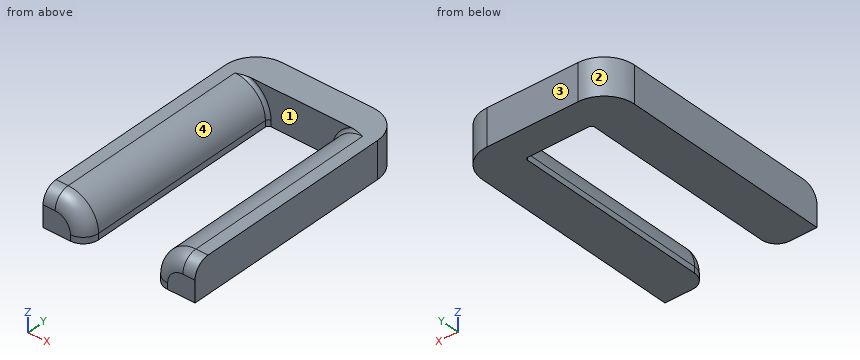
```python
from build123d import *

# Parameters (mm, degrees)
F0_W         = 50
F0_H         = 12
F1_DEPTH     = 10
F2_W         = 14
F2_H         = 12
F3_DEPTH     = 70
F4_R         = 10
F5_R         = 5
F6_T1_DEPTH  = 2
F6_T6_ANGLE  = 132.9890967712
F6_T12_ANGLE = 132.9890967712
F7_R         = 10


# Not quite as in the source:
# - a fillet or chamfer that OpenCascade refuses, or shapes differently, is made with other operations: its cross-section is extruded or revolved along the edge and cut away or added


with BuildPart() as f1:
    # F0 (on Front) → F1 (new body)
    with BuildSketch(Plane.XZ):
        with Locations((25, 6)):
            Rectangle(F0_W, F0_H)
    extrude(amount=F1_DEPTH)

    # F2 (on face) → F3 (join)
    with BuildSketch(Plane.XZ.offset(10)):
        with Locations((7, 6)):
            Rectangle(F2_W, F2_H)
        with Locations((43, 6)):
            Rectangle(F2_W, F2_H)
    extrude(amount=F3_DEPTH)

    # F4
    f4_edges = [f1.edges().sort_by_distance(p)[0] for p in [
        (14, -45, 12),
        (36, -45, 12),
    ]]
    fillet(f4_edges, radius=F4_R)

    # F5
    f5_edges = [f1.edges().sort_by_distance(p)[0] for p in [
        (11.071068, -80, 9.071068),
        (38.928932, -80, 9.071068),
        (48, -80, 12),
        (36, -80, 1),
        (2, -80, 12),
        (14, -80, 1),
    ]]
    fillet(f5_edges, radius=F5_R)

    # F6: fillet of radius 1 on 4 edges, made by hand

    # F6_s2 → F6_t1 (join)
    with BuildSketch(Plane.XY):
        with BuildLine():
            ThreePointArc((14, -11), (14.2928932188, -10.2928932188), (15, -10))
            Line((15, -10), (14, -10))
            Line((14, -10), (14, -11))
        make_face()
        with BuildLine():
            ThreePointArc((35, -10), (35.7071067812, -10.2928932188), (36, -11))
            Line((36, -11), (36, -10))
            Line((36, -10), (35, -10))
        make_face()
    extrude(amount=F6_T1_DEPTH)


with BuildPart() as f6_tool4:
    # F6_s5 → F6_t6 (revolve)
    with BuildSketch(Plane.XY.offset(2)):
        with BuildLine():
            ThreePointArc((15, -10), (14.2928932188, -10.2928932188), (14, -11))
            Line((14, -11), (14, -10))
            Line((14, -10), (15, -10))
        make_face()
    revolve(axis=Axis((4, -10, 2), (0, -1, 0)), revolution_arc=F6_T6_ANGLE)

    split(bisect_by=Plane.XY.offset(12), keep=Keep.BOTTOM)

    split(bisect_by=Plane.YZ, keep=Keep.TOP)


with BuildPart() as f1_1:
    add(f1.part)

    # F6_t3: union F6_tool4
    add(f6_tool4.part)


with BuildPart() as f6_tool10:
    # F6_s11 → F6_t12 (revolve)
    with BuildSketch(Plane.XY.offset(2)):
        with BuildLine():
            ThreePointArc((35, -10), (35.7071067812, -10.2928932188), (36, -11))
            Line((36, -11), (36, -10))
            Line((36, -10), (35, -10))
        make_face()
    revolve(axis=Axis((46, -10, 2), (0, 1, 0)), revolution_arc=F6_T12_ANGLE)

    split(bisect_by=Plane.YZ.offset(50), keep=Keep.BOTTOM)

    split(bisect_by=Plane.XY.offset(12), keep=Keep.BOTTOM)


with BuildPart() as f1_2:
    add(f1_1.part)

    # F6_t9: union F6_tool10
    add(f6_tool10.part)

    # F7
    f7_edges = [f1_2.edges().sort_by_distance(p)[0] for p in [
        (50, 0, 6),
        (0, 0, 6),
    ]]
    fillet(f7_edges, radius=F7_R)


solid = f1_2.part
```
Design review of the part built by this model. Coordinates are the model's own, in mm. Face numbers are marked on the shaded views. Coordinates: 2 decimals unless noted, no trailing zeros. Order: outer loops, then holes, each group sorted by start corner. A loop starts at its lowest first (then second) coordinate and runs counter-clockwise, first axis right, second up. Notation, with made-up numbers: (5.25, 27.25) - (10.25, 27.25) arc R12 ccw to (10.25, 39.25) - close; hole circle Ø1 at (22.25, -37). An arc over 180 degrees is marked (long way). One line per question, with ' | ' between items.
Q1. Consider section A-A, the plane y = -40. Give the boundary of the cut face in (x, z), then the cut area to 3 significant figures.
Answer key:
outline: (0, 0) - (14, 0) - (14, 2) arc R10 ccw to (4, 12) - (0, 12) - close; (36, 0) - (50, 0) - (50, 12) - (46, 12) arc R10 ccw to (36, 2) - close | area: 293 mm2
Q2. Consider section C-C, the plane y = -7. Give the boundary of the cut face in (x, z).
Answer key:
outline: (0.46, 0) - (49.54, 0) - (49.54, 12) - (0.46, 12) - close
Q3. To check wall thickness, follow line 1 along X through (y, z) = (-28.5, 10); line 2 along X through (y, z) = (-65, 1.5); line 3 along Y through (x, z) = (40, 11.5). State the ranges of each line that lie inside material, in increasing order.
Answer key:
line 1: x = 0 to 10, 40 to 50 | line 2: x = 0 to 14, 36 to 50 | line 3: y = -10 to 0
Q4. Consider section B-B, the plane x = 26. Give the boundary of the cut face in (y, z), then the cut area to 3 significant figures.
Answer key:
outline: (-10, 0) - (0, 0) - (0, 12) - (-10, 12) - close | area: 120 mm2
Q5. The part is to be moulded in two halves that separate along X. For the marked faces 1, 2, 3 and 4, say which applies: +X half, -X half, draft (parallel to the pull), parting line (faces both ways), or undercut.
Answer key:
face 1: undercut | face 2: -X half | face 3: draft | face 4: undercut
Q6. Clearance check with flat-ended pins moving along their axes: pin 1 Ø8 at (x, y) = (13, -14.5) entering from +Z; pin 2 Ø2 at (x, y) = (6.5, -45.5) entering from +Z. State where each tip first meets the part, or that it passes through.
Answer key:
pin 1: stops at z = 10.66 | pin 2: stops at z = 11.89
